Design review of the part built by this model. Coordinates are the model's own, in mm. Face numbers are marked on the shaded views. A direction names the side the tool comes from. Give positions to 0.01 mm unless a question says otherwise; leave off trailing zeros. Order: outer loops, then holes, each group sorted by start corner. A loop starts at its lowest first (then second) coordinate and runs counter-clockwise, first axis right, second up. Notation, with made-up numbers: (43, 75.25) -> (60, 75.25) arc R20 ccw to (60, 87.25) -> close; hole circle Ø6 at (40, 87.5). An arc over 180 degrees is marked (long way). Use a Markdown table: item, result. Add a question column.
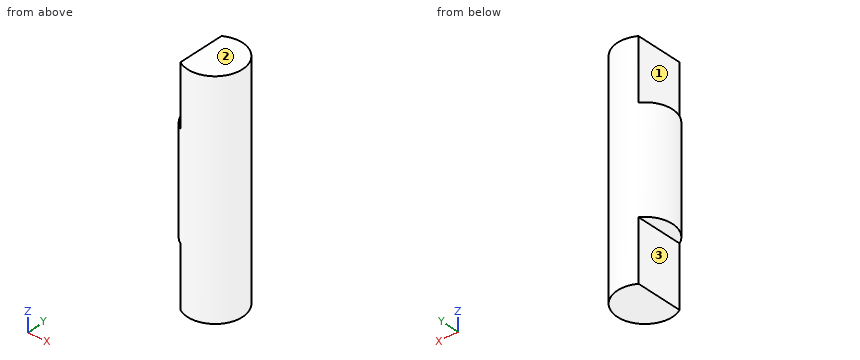
```python
from build123d import *

# Parameters (mm, degrees)
SKETCH2_R           = 1.95
BOSS_EXTRUDE1_DEPTH = 8
CUT_EXTRUDE1_DEPTH  = 4.3


with BuildPart() as part:
    # Sketch2 → Boss-Extrude1 (new body, symmetric)
    with BuildSketch(Plane.XY):
        Circle(SKETCH2_R)
    extrude(amount=BOSS_EXTRUDE1_DEPTH, both=True)

    # Sketch4 → Cut-Extrude1 (cut)
    with BuildSketch(Plane(origin=(0, 0, -8), x_dir=(-1, 0, 0), z_dir=(0, 0, -1))):
        with BuildLine():
            Line((1, 1.674066904), (1, -1.674066904))
            ThreePointArc((1, -1.674066904), (1.95, 0), (1, 1.674066904))
        make_face()
    cut_extrude1 = extrude(amount=-CUT_EXTRUDE1_DEPTH, mode=Mode.SUBTRACT)

    # Mirror1: Cut-Extrude1 across plane
    add(cut_extrude1.mirror(Plane.XY), mode=Mode.SUBTRACT)


solid = part.part
```
1) For L1, parallel to X at y = -0.1, z = -1.25; L2, parallel to Y at x = 0.4, z = 2.75; L3, parallel to X at y = -0.75, z = -3.25, list the stretches that pass through material, from the lowest coordinate up. Write a range as [from, to].
2) Insertion check: pin 1 (2 mm diameter, centred on y = -1, z = -5.5, fed in from -X); pin 2 (1.5 mm diameter, centred on y = 1.5, z = 3.5, fed in from -X); pin 3 (1 mm diameter, centred on y = 1, z = -2.5, fed in from +X). Each pin has a flat end and moves straight along its axis. Give the tip position at first contact, or say it passes through.
3) Add section C-C (x = 0.65). Give the boundary of the cut face in (y, z).
4) Add section A-A (y = 0). Give the boundary of the cut face in (x, z).
5) Add section B-B (z = -3.5). Give the boundary of the cut face in (x, y).
6) Add section D-D (x = -1.25). Give the boundary of the cut face in (y, z), then the cut area to 3 significant figures.
7) Machinability: for the marked faces 1, 2 and 3, which of the approach directions +Z, -Z, +X, -X, +Y, -Y give a long, thin tool a straight path to every point of the face, cutting with its end or side? Answer none if there is none.
Worked answers:
| question | item | result |
|---|---|---|
| 1 | L1 | [-1.95, 1.95] |
| 1 | L2 | [-1.91, 1.91] |
| 1 | L3 | [-1.8, 1.8] |
| 2 | pin 1 | x = -1 |
| 2 | pin 2 | x = -1.8 |
| 2 | pin 3 | x = 1.88 |
| 3 | outline | (-1.84, -8) -> (1.84, -8) -> (1.84, 8) -> (-1.84, 8) -> close |
| 4 | outline | (-1.95, -3.7) -> (-1, -3.7) -> (-1, -8) -> (1.95, -8) -> (1.95, 8) -> (-1, 8) -> (-1, 3.7) -> (-1.95, 3.7) -> close |
| 5 | outline | circle Ø3.9 at (0, 0) |
| 6 | outline | (-1.5, -3.7) -> (1.5, -3.7) -> (1.5, 3.7) -> (-1.5, 3.7) -> close |
| 6 | area | 22.2 mm^2 |
| 7 | face 1 | +Z, -X, +Y, -Y |
| 7 | face 2 | +Z, +X, -X, +Y, -Y |
| 7 | face 3 | -Z, -X, +Y, -Y |
